For this review, use the dimensioned drawing (mm, ordinates from the lowest corner) and the shaded views. A direction names the side the tool comes from. Round coordinates to 2 decimals unless told otherwise and drop trailing zeros. Order: outer loops, then holes, each group sorted by start corner. A loop starts at its lowest first (then second) coordinate and runs counter-clockwise, first axis right, second up. Notation, with made-up numbers: (-21.75, 80.25) - (10.25, 80.25) arc R23 ccw to (10.25, 95.25) - close; hole circle Ø2 at (31.5, 71.25). An arc over 180 degrees is marked (long way). Write item = value, one per line.
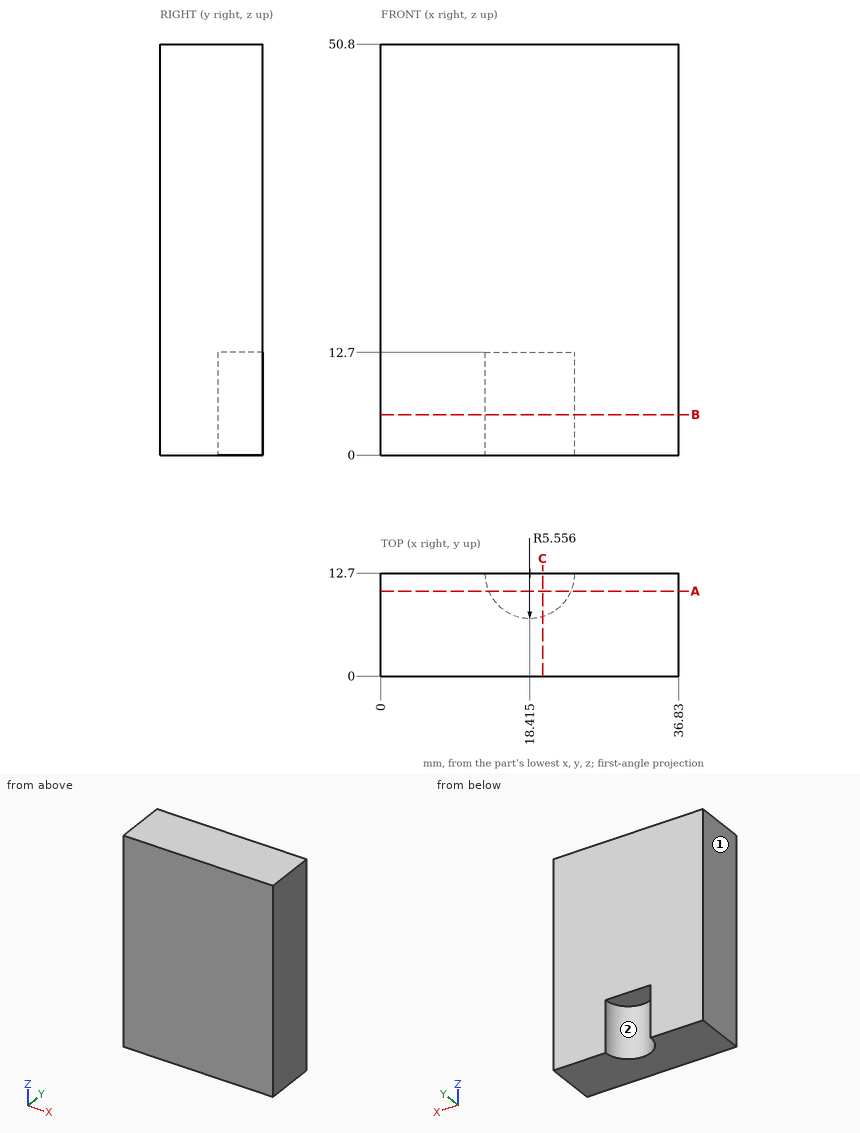
Item 1: Take a section at A-A, the plane y = 10.5. State the section outline as (x, z) points, and give its area (3 significant figures).
Data:
outline = (0, 0) - (13.31, 0) - (13.31, 12.7) - (23.52, 12.7) - (23.52, 0) - (36.83, 0) - (36.83, 50.8) - (0, 50.8) - close
area = 1,740 mm2
Item 2: Take a section at B-B, the plane z = 5. State the section outline as (x, y) points (1 decimal).
Data:
outline = (0, 0) - (36.8, 0) - (36.8, 12.7) - (24, 12.7) arc R5.6 cw to (12.9, 12.7) - (0, 12.7) - close
Item 3: For the marked faces 1 and 2, list the 3-axis set-ups (+Z, -Z, +X, -X, +Y, -Y) from which the entire face can be reached by the end or side of a thin tool; tool diameter is ignored.
Data:
face_1 = +Z, -Z, -X, +Y, -Y
face_2 = -Z, +Y
Item 4: For line 1 along Y through (x, z) = (19, 10) (1 decimal); line 2 along X through (y, z) = (11.75, 7); line 3 along X through (y, z) = (11.25, 12), list the stretches that pass through material, from the lowest coordinate up. Write a range as [from, to].
Data:
line_1 = [0, 7.2]
line_2 = [0, 12.94], [23.89, 36.83]
line_3 = [0, 13.05], [23.78, 36.83]
Item 5: Take a section at C-C, the plane x = 20. State the section outline as (y, z) points (1 decimal).
Data:
outline = (0, 0) - (7.4, 0) - (7.4, 12.7) - (12.7, 12.7) - (12.7, 50.8) - (0, 50.8) - close
Item 6: Insertion check: P1, Ø8, axis at x = 10.5, z = 18.5, coming from the -Y side. The pin has a flat end and moves straight along its axis. Give the tip position at first contact, or say it passes through.
Data:
P1 = 0
